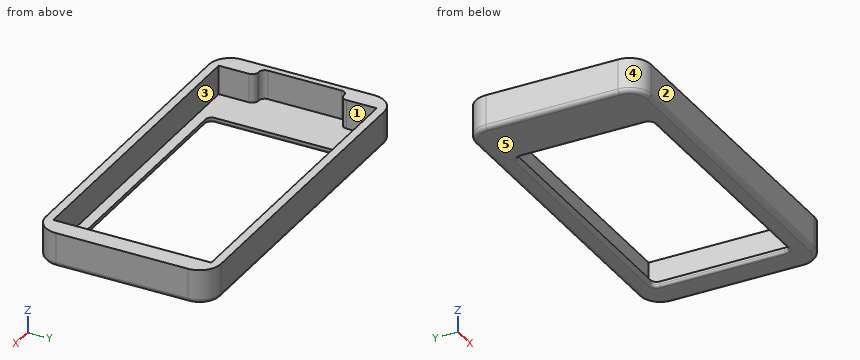
```python
from build123d import *

# Parameters (mm, degrees)
SKETCH1_W           = 81
SKETCH1_H           = 41
BOSS_EXTRUDE1_DEPTH = 8
SKETCH2_W           = 72
SKETCH2_H           = 37
CUT_EXTRUDE1_DEPTH  = 6.8
SKETCH3_W           = 3
SKETCH3_H           = 20
CUT_EXTRUDE2_DEPTH  = 6.8
SKETCH4_W           = 60.6
SKETCH4_H           = 32
CUT_EXTRUDE3_DEPTH  = 6.4
FILLET1_R           = 1.4
FILLET2_R           = 5
FILLET3_R           = 0.6
FILLET4_R           = 1


with BuildPart() as part:
    # Sketch1 → Boss-Extrude1 (new body)
    with BuildSketch(Plane.XY):
        with Locations((40.5, 20.5)):
            Rectangle(SKETCH1_W, SKETCH1_H)
    extrude(amount=BOSS_EXTRUDE1_DEPTH)

    # Sketch2 → Cut-Extrude1 (cut)
    with BuildSketch(Plane.XY.offset(8)):
        with Locations((40.5, 20.5)):
            Rectangle(SKETCH2_W, SKETCH2_H)
    extrude(amount=-CUT_EXTRUDE1_DEPTH, mode=Mode.SUBTRACT)

    # Sketch3 → Cut-Extrude2 (cut)
    with BuildSketch(Plane.XY.offset(8)):
        with Locations((3, 20.5)):
            Rectangle(SKETCH3_W, SKETCH3_H)
    extrude(amount=-CUT_EXTRUDE2_DEPTH, mode=Mode.SUBTRACT)

    # Sketch4 → Cut-Extrude3 (cut)
    with BuildSketch(Plane.XY.offset(1.2)):
        with Locations((43.8, 20.5)):
            Rectangle(SKETCH4_W, SKETCH4_H)
    extrude(amount=-CUT_EXTRUDE3_DEPTH, mode=Mode.SUBTRACT)

    # Fillet1
    fillet1_edges = [part.edges().sort_by_distance(p)[0] for p in [
        (4.5, 30.5, 4.6),
        (4.5, 10.5, 4.6),
        (1.5, 10.5, 4.6),
        (1.5, 30.5, 4.6),
        (13.5, 4.5, 0.6),
        (13.5, 36.5, 0.6),
        (74.1, 36.5, 0.6),
        (74.1, 4.5, 0.6),
    ]]
    fillet(fillet1_edges, radius=FILLET1_R)

    # Fillet2
    fillet2_edges = [part.edges().sort_by_distance(p)[0] for p in [
        (0, 41, 4),
        (81, 41, 4),
        (81, 0, 4),
        (0, 0, 4),
    ]]
    fillet(fillet2_edges, radius=FILLET2_R)

    # Fillet3
    fillet3_edges = [part.edges().sort_by_distance(p)[0] for p in [
        (74.1, 20.5, 0),
        (43.8, 4.5, 0),
        (13.5, 20.5, 0),
        (43.8, 36.5, 0),
        (73.689949494, 4.910050506, 0),
        (13.910050506, 4.910050506, 0),
        (13.910050506, 36.089949494, 0),
        (73.689949494, 36.089949494, 0),
    ]]
    fillet(fillet3_edges, radius=FILLET3_R)

    # Fillet4
    fillet4_edges = [part.edges().sort_by_distance(p)[0] for p in [
        (40.5, 0, 0),
        (0, 20.5, 0),
        (40.5, 41, 0),
        (81, 20.5, 0),
        (1.464466094, 39.535533906, 0),
        (79.535533906, 39.535533906, 0),
        (79.535533906, 1.464466094, 0),
        (1.464466094, 1.464466094, 0),
    ]]
    fillet(fillet4_edges, radius=FILLET4_R)


solid = part.part
```
Check sheet for the modelled part. Datum: model origin and axes. Units: mm. Face numbers are marked on the shaded views. A direction names the side the tool comes from. Round coordinates to 2 decimals unless told otherwise and drop trailing zeros. Loops run counter-clockwise (first coordinate to the right, second up) from the corner with the lowest first, then second, coordinate; pieces in that order, holes last. Notation, with made-up numbers: (60.5, 23.25) - (97.5, 23.25) arc R20 cw to (97.5, 41.25) - close; hole circle Ø6 at (78, 85.25). An arc over 180 degrees is marked (long way). Answer as a JSON object with one key per item and string values. Group by question number.
Q1. Sectioned sample at A-A, the plane x = 57. Enter the section's corners in (y, z), plus the area to 3 significant figures.
Q2. Gauge pin test, flat end, axial feed: P1, Ø10, axis at x = 29, y = 32, coming from the +Z side. Record the tip position at first contact, or that the pin passes through.
Q3. Sectioned sample at C-C, the plane y = 20.5. Enter the section's corners in (x, z), plus the area to 3 significant figures.
Q4. Mould release check, pull along Y, two halves, no side actions. Record for the marked faces 3, 4 and 5: released by +Y, released by -Y, zero draft, split by the parting line, or undercut.
Q5. Sectioned sample at B-B, the plane z = 6.5. Enter the section's corners in (x, y), plus the area to 3 significant figures.
Q6. Scan lines: line 1 along Y through (x, z) = (8, 1.75); line 2 along X through (y, z) = (32.5, 5.75); line 3 along X through (y, z) = (22.5, 2). Record each from-to range of solid material in increasing order. Write a range as [from, to].
Q7. Set-up check for the marked faces 1 and 2: record each of +Z, -Z, +X, -X, +Y, -Y from which the full face is reachable in a straight line by a thin tool's end or side.
Solution:
{
 "1": {"outline": "(0, 1) arc R1 ccw to (1, 0) - (3.9, 0) arc R0.6 ccw to (4.5, 0.6) - (4.5, 1.2) - (2, 1.2) - (2, 8) - (0, 8) - close; (36.5, 0.6) arc R0.6 ccw to (37.1, 0) - (40, 0) arc R1 ccw to (41, 1) - (41, 8) - (39, 8) - (39, 1.2) - (36.5, 1.2) - close", "area": "37.4 mm²"},
 "2": {"P1": "stops at z = 1.2"},
 "3": {"outline": "(0, 1) arc R1 ccw to (1, 0) - (12.9, 0) arc R0.6 ccw to (13.5, 0.6) - (13.5, 1.2) - (1.5, 1.2) - (1.5, 8) - (0, 8) - close; (74.1, 0.6) arc R0.6 ccw to (74.7, 0) - (80, 0) arc R1 ccw to (81, 1) - (81, 8) - (76.5, 8) - (76.5, 1.2) - (74.1, 1.2) - close", "area": "64.7 mm²"},
 "4": {"face 3": "undercut", "face 4": "released by -Y", "face 5": "zero draft"},
 "5": {"outline": "(0, 5) arc R5 ccw to (5, 0) - (76, 0) arc R5 ccw to (81, 5) - (81, 36) arc R5 ccw to (76, 41) - (5, 41) arc R5 ccw to (0, 36) - close; hole (1.5, 11.9) arc R1.4 ccw to (2.9, 10.5) - (3.1, 10.5) arc R1.4 cw to (4.5, 9.1) - (4.5, 2) - (76.5, 2) - (76.5, 39) - (4.5, 39) - (4.5, 31.9) arc R1.4 cw to (3.1, 30.5) - (2.9, 30.5) arc R1.4 ccw to (1.5, 29.1) - close", "area": "576 mm²"},
 "6": {"line 1": "y = [0, 2], [39, 41]", "line 2": "x = [0, 4.5], [76.5, 81]", "line 3": "x = [0, 1.5], [76.5, 81]"},
 "7": {"face 1": "+Z", "face 2": "+Z, -Z, +X, -X, -Y"}
}
